```python
from build123d import *

# Parameters (mm, degrees)
BOSS_EXTRUDE1_DEPTH = 1.5
FILLET1_R           = 50


with BuildPart() as part:
    # Sketch2 → Boss-Extrude1 (new, symmetric)
    with BuildSketch(Plane.XY):
        Polygon((15, 24), (30, 24), (30, 36), (25, 36), (25, 39), (-25, 39), (-25, 36), (-30, 36), (-30, 24), (-15, 24), (-15, -24), (-10, -24), (-10, -27), (10, -27), (10, -24), (15, -24), align=None)
    extrude(amount=BOSS_EXTRUDE1_DEPTH, both=True)

    # Fillet1
    # the kernel refuses this fillet: 50 mm, written as the material it adds along each edge
    with BuildSketch(Plane(origin=(-15, 24, -1.5), x_dir=(0, -1, 0), z_dir=(0, 0, 1))) as fillet1_piece_1:
        with BuildLine():
            CenterArc((35.707142143, -50), FILLET1_R, 90, 45.572995999)
            Line((0, -15), (0, 0))
            Line((0, 0), (35.707142143, 0))
        make_face()
    extrude(amount=3)
    with BuildSketch(Plane(origin=(15, 24, 1.5), x_dir=(1, 0, 0), z_dir=(0, 0, -1))) as fillet1_piece_2:
        with BuildLine():
            CenterArc((50, 35.707142143), FILLET1_R, 180, 45.572995999)
            Line((0, 35.707142143), (0, 0))
            Line((0, 0), (15, 0))
        make_face()
    extrude(amount=3)


solid = part.part
```
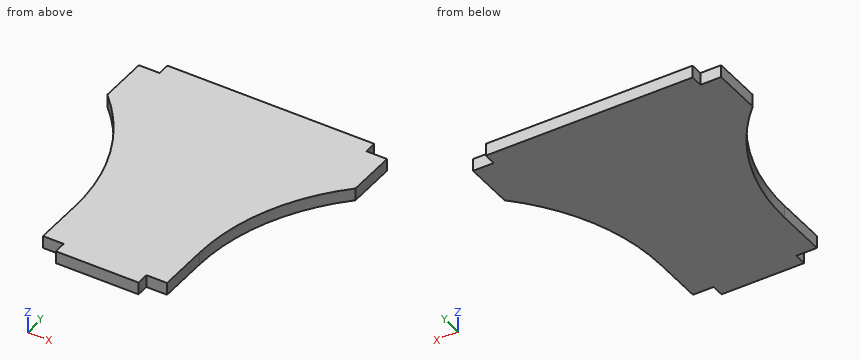
Can you work these out from the model? Positions are in its coordinate system, mm. Coordinates: 2 decimals unless noted, no trailing zeros. Write each loop counter-clockwise with the first axis right and the second up, starting at its lowest first coordinate (ties: lowest second). Pieces come first, ordered by that corner, then holes. Notation, with made-up numbers: (19.5, -6.5) - (46.5, -6.5) arc R14 ccw to (46.5, 1.5) - close; hole circle Ø7 at (58.25, 19.25). An arc over 180 degrees is marked (long way). Return JSON: item names as keys, results as strings.
Q1. If we section it at A-A (z = 0.8): Please give me the cut outline in (x, y), then the cut area to 3 significant figures.
Computed values:
{"outline": "(-30, 24) arc R50 cw to (-15, -11.71) - (-15, -24) - (-10, -24) - (-10, -27) - (10, -27) - (10, -24) - (15, -24) - (15, -11.71) arc R50 cw to (30, 24) - (30, 36) - (25, 36) - (25, 39) - (-25, 39) - (-25, 36) - (-30, 36) - close", "area": "2,700 mm2"}
Q2. If we section it at C-C (y = 23): Please give me the cut outline in (x, z).
Computed values:
{"outline": "(-29.01, -1.5) - (29.01, -1.5) - (29.01, 1.5) - (-29.01, 1.5) - close"}
Q3. I'm going to push flat-ended pins straight in: pin 1 Ø1.5 at (y, z) = (37.5, -0.5) entering from +X; pin 2 Ø1.5 at (y, z) = (-21, 0) entering from +X; pin 3 Ø0.9 at (y, z) = (37.5, -0.5) entering from -X. Where does each tip first touch, or does it pass through?
Computed values:
{"pin 1": "stops at x = 25", "pin 2": "stops at x = 15", "pin 3": "stops at x = -25"}
Q4. If we section it at B-B (x = -22): Please give me the cut outline in (y, z), then the cut area to 3 significant figures.
Computed values:
{"outline": "(13.81, -1.5) - (39, -1.5) - (39, 1.5) - (13.81, 1.5) - close", "area": "75.6 mm2"}
Q5. Please list where these lines run through material, in increasing order: L1, parallel to Y at x = 14.5, z = -0.9; L2, parallel to Y at x = 22, z = 0.9; L3, parallel to X at y = -23, z = 0.95. Write a range as from..to.
Computed values:
{"L1": "y = -24..39", "L2": "y = 13.81..39", "L3": "x = -15..15"}
